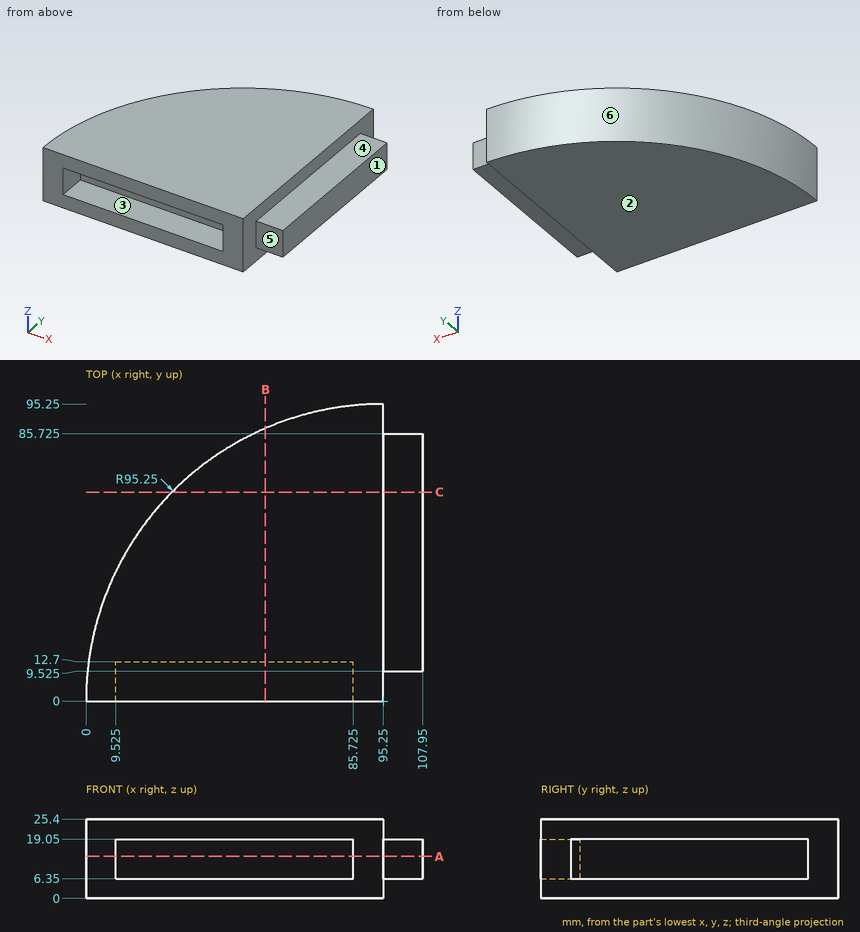
Print and shaded views of the part. All mm, measured from the part's lowest x, y and z. A direction names the side the tool comes from. Give positions to 0.01 mm unless a question says otherwise; leave off trailing zeros. Write each loop counter-clockwise with the first axis right and the second up, starting at its lowest first coordinate (ties: lowest second). Pieces come first, ordered by that corner, then holes. Notation, with made-up numbers: (77, 65.25) -> (136, 65.25) arc R36 cw to (136, 100.25) -> close; hole circle Ø3 at (38.25, 43.25). An arc over 180 degrees is marked (long way). Use CSV: the item, a comma, the result in double quotes. Start each with the question number.
1) Drill centre lines: L1, parallel to Z at x = 96, y = 62; L2, parallel to X at y = 72, z = 11.5; L3, parallel to X at y = 73, z = 22.75. Where is each one in solid material? Low to high.
2) Two-plate mould, pull along X, no slides. Class the marked faces 1, 2 and 3: released by +X, released by -X, zero draft, split by the parting line, or undercut.
3) Pin check, flat tips, straight feed: P1, Ø4, axis at x = 101, z = 10, coming from the +Y side (3 decimals); P2, Ø4, axis at x = 60, z = 9, coming from the +Y side; P3, Ø10, axis at x = 104.5, y = 35, coming from the +Z side. Stop position of each tip, or through.
4) Cut at A-A on z = 13.5. List the corners of the cut face in (x, y) (3 decimals), plus the area to 3 significant figures.
5) Cut at B-B on x = 57.5. List the corners of the cut face in (y, z).
6) Cut at C-C on y = 67. List the corners of the cut face in (x, z), plus the area to 3 significant figures.
7) Tool access for the marked faces 4, 5 and 6: list every direction of +Z, -Z, +X, -X, +Y, -Y with a clear straight run to the whole face (end or side of a thin tool).
Final values:
1,L1,"z = 6.35 to 19.05"
1,L2,"x = 32.89 to 107.95"
1,L3,"x = 34.07 to 95.25"
2,face 1,"released by +X"
2,face 2,"zero draft"
2,face 3,"undercut"
3,P1,"stops at y = 85.725"
3,P2,"stops at y = 89.26"
3,P3,"stops at z = 19.05"
4,outline,"(0, 0) -> (9.525, 0) -> (9.525, 12.7) -> (85.725, 12.7) -> (85.725, 0) -> (95.25, 0) -> (95.25, 9.525) -> (107.95, 9.525) -> (107.95, 85.725) -> (95.25, 85.725) -> (95.25, 95.25) arc R95.25 ccw to start"
4,area,"7,130 mm2"
5,outline,"(0, 0) -> (87.45, 0) -> (87.45, 25.4) -> (0, 25.4) -> (0, 19.05) -> (12.7, 19.05) -> (12.7, 6.35) -> (0, 6.35) -> close"
6,outline,"(27.55, 0) -> (95.25, 0) -> (95.25, 6.35) -> (107.95, 6.35) -> (107.95, 19.05) -> (95.25, 19.05) -> (95.25, 25.4) -> (27.55, 25.4) -> close"
6,area,"1,880 mm2"
7,face 4,"+Z, +X, +Y, -Y"
7,face 5,"+Z, -Z, +X, -Y"
7,face 6,"+Z, -Z, -X, +Y"
